For this review, take the finished solid that the model builds, in its own axes (mm). Face numbers are marked on the shaded views. A direction names the side the tool comes from. Round coordinates to 2 decimals unless told otherwise and drop trailing zeros. Loops run counter-clockwise (first coordinate to the right, second up) from the corner with the lowest first, then second, coordinate; pieces in that order, holes last. Notation, with made-up numbers: M 60.5,-8 L 105.5,-8 A9 ccw 105.5,9 Z; hole C -10.75,-25.5 d5. An arc over 180 degrees is marked long. Write item = value, one per line. Start each with the question number.
```python
from build123d import *

# Parameters (mm, degrees)
SKETCH1_R           = 45
SKETCH1_R_2         = 11.5
BOSS_EXTRUDE1_DEPTH = 14
SKETCH3_R           = 3
SKETCH6_R           = 3
CUT_EXTRUDE3_DEPTH  = 3
SKETCH7_R           = 1.75
CUT_EXTRUDE4_DEPTH  = 13
SKETCH8_W           = 21.8
SKETCH8_H           = 42.5
CUT_EXTRUDE7_DEPTH  = 9.5
SKETCH9_R           = 42.5
SKETCH9_R_2         = 40.5
BOSS_EXTRUDE2_DEPTH = 10


with BuildPart() as part:
    # Sketch1 → Boss-Extrude1 (new body)
    with BuildSketch(Plane(origin=(0, 0, 0), x_dir=(1, 0, 0), z_dir=(0, 1, 0))):
        with Locations(Location((0, 0, 0), (0, 0, 270))):
            Circle(SKETCH1_R)
        with Locations(Location((0, 0, 0), (0, 0, 270))):
            Circle(SKETCH1_R_2, mode=Mode.SUBTRACT)
    extrude(amount=BOSS_EXTRUDE1_DEPTH)

    # Sketch3 → Cut-Revolve1 (revolve, cut)
    with BuildSketch(Plane.XY, mode=Mode.PRIVATE) as cut_revolve1_sk:
        with Locations((-28, 14)):
            Circle(SKETCH3_R)
    revolve(cut_revolve1_sk.sketch.rotate(Axis((0, 14, 0), (0, -1, 0)), 270), axis=Axis((0, 14, 0), (0, -1, 0)), mode=Mode.SUBTRACT)

    # Sketch6 → Cut-Extrude3 (cut)
    with BuildSketch(Plane(origin=(0, 14, 0), x_dir=(1, 0, 0), z_dir=(0, 1, 0))):
        with Locations(Location((-4.9, -34.65, 0), (0, 0, 270))):
            Circle(SKETCH6_R)
        with Locations(Location((4.9, -34.65, 0), (0, 0, 270))):
            Circle(SKETCH6_R)
        with Locations(Location((-4.9, 13.85, 0), (0, 0, 270))):
            Circle(SKETCH6_R)
        with Locations(Location((4.9, 13.85, 0), (0, 0, 270))):
            Circle(SKETCH6_R)
    extrude(amount=-CUT_EXTRUDE3_DEPTH, mode=Mode.SUBTRACT)

    # Sketch7 → Cut-Extrude4 (cut)
    with BuildSketch(Plane.XZ):
        with Locations(Location((4.9, 34.65, 0), (0, 0, 270))):
            Circle(SKETCH7_R)
        with Locations(Location((-4.9, 34.65, 0), (0, 0, 270))):
            Circle(SKETCH7_R)
        with Locations(Location((4.9, -13.85, 0), (0, 0, 270))):
            Circle(SKETCH7_R)
        with Locations(Location((-4.9, -13.85, 0), (0, 0, 270))):
            Circle(SKETCH7_R)
    extrude(amount=-CUT_EXTRUDE4_DEPTH, mode=Mode.SUBTRACT)

    # Sketch8 → Cut-Extrude7 (cut)
    with BuildSketch(Plane.XZ):
        with Locations((0, 10.4)):
            Rectangle(SKETCH8_W, SKETCH8_H)
    extrude(amount=-CUT_EXTRUDE7_DEPTH, mode=Mode.SUBTRACT)

    # Sketch9 → Boss-Extrude2 (add)
    with BuildSketch(Plane.XZ):
        with Locations(Location((0, 0, 0), (0, 0, 90))):
            Circle(SKETCH9_R)
        with Locations(Location((0, 0, 0), (0, 0, 270))):
            Circle(SKETCH9_R_2, mode=Mode.SUBTRACT)
    extrude(amount=BOSS_EXTRUDE2_DEPTH)


solid = part.part
```
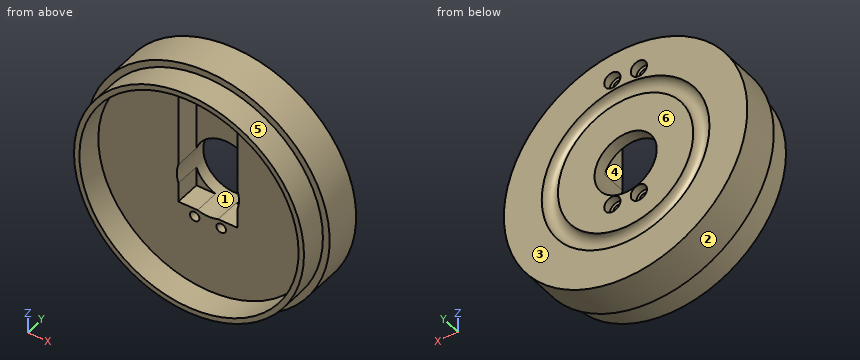
(1) Add section D-D on z = 34.65. Write out the cut boundary in (x, y).
(2) Wall thickness on L1, parallel to X at y = 12.8, z = -13.85; L2, parallel to X at y = 8.25, z = 34.65; L3, parallel to Z at x = 12, y = -7.5: over which ranges is each line inside the solid? List them lowest first.
(3) Add section C-C on x = 0. Write out the cut boundary in (y, z).
(4) For pin 1 Ø3 at (x, y) = (15.5, -5) entering from -Z; pin 2 Ø5 at (x, z) = (-4.9, -13.85) entering from -Y; pin 3 Ø5 at (x, y) = (25, 3) entering from -Z, all flat-tipped, find the tip position at first contact; note any pin that passes through.
(5) Tool access review of the marked faces 5 and 6: name each direction out of +Z, -Z, +X, -X, +Y, -Y from which nothing blocks a thin tool from reaching the whole face with its end or side.
(6) Draft analysis for pull direction X (two halves, no side actions). For the marked faces 1, 2, 3 and 4, state which applies: +X half, -X half, draft (parallel to the pull), parting line (faces both ways), or undercut.
(7) Add section A-A on z = 0. Write out the cut boundary in (x, y).
(8) Add section B-B on y = 5. Write out the cut boundary in (x, z), and give its area (3 significant figures).
Answer sheet:
q1.outline = M -28.71,0 L -24.61,0 L -24.61,-10 L -20.97,-10 L -20.97,0 L -6.65,0 L -6.65,11 L -7.9,11 L -7.9,14 L -28.71,14 Z; M -3.15,0 L 3.15,0 L 3.15,11 L 1.9,11 L 1.9,14 L -1.9,14 L -1.9,11 L -3.15,11 Z; M 6.65,0 L 20.97,0 L 20.97,-10 L 24.61,-10 L 24.61,0 L 28.71,0 L 28.71,14 L 7.9,14 L 7.9,11 L 6.65,11 Z
q2.L1 = -42.82 to -27.45, -21.11 to -7.9, -1.9 to 1.9, 7.9 to 21.11, 27.45 to 42.82
q2.L2 = -28.71 to -6.65, -3.15 to 3.15, 6.65 to 28.71
q2.L3 = -40.77 to -38.68, 38.68 to 40.77
q3.outline = M -10,-42.5 L 0,-42.5 L 0,-45 L 14,-45 L 14,-31 A3 cw 14,-25 L 14,-11.5 L 0,-11.5 L 0,-40.5 L -10,-40.5 Z; M -10,40.5 L 0,40.5 L 0,31.65 L 9.5,31.65 L 9.5,11.5 L 14,11.5 L 14,25 A3 cw 14,31 L 14,45 L 0,45 L 0,42.5 L -10,42.5 Z
q4.pin_1 = -40.13
q4.pin_2 = 0
q4.pin_3 = -38.97
q5.face_5 = -Y
q5.face_6 = +Z, -Z, +X, -X, +Y
q6.face_1 = undercut
q6.face_2 = parting line
q6.face_3 = draft
q6.face_4 = undercut
q7.outline = M -45,0 L -42.5,0 L -42.5,-10 L -40.5,-10 L -40.5,0 L -11.5,0 L -11.5,14 L -25,14 A3 cw -31,14 L -45,14 Z; M 11.5,0 L 40.5,0 L 40.5,-10 L 42.5,-10 L 42.5,0 L 45,0 L 45,14 L 31,14 A3 cw 25,14 L 11.5,14 Z
q8.outline = C 0,0 d90; hole M -10.9,-10.85 L -3.81,-10.85 A11.5 ccw 3.81,-10.85 L 10.9,-10.85 L 10.9,-3.67 A11.5 ccw 10.9,3.67 L 10.9,31.65 L -10.9,31.65 L -10.9,3.67 A11.5 ccw -10.9,-3.67 Z; hole C -4.9,-13.85 d3.5; hole C -4.9,34.65 d3.5; hole C 4.9,-13.85 d3.5; hole C 4.9,34.65 d3.5
q8.area = 5,390 mm²
